```python
from build123d import *

# Parameters (mm, degrees)
F0_W          = 12
F0_H          = 23
F1_DEPTH      = 23.35
F2_W          = 12
F2_H          = 2.3
F3_DEPTH      = 5
F3_DEPTH_BACK = 28
F5_DEPTH      = 3.8
F6_R          = 2.325
F7_DEPTH      = 2.5
F9_DEPTH      = 25
F11_DEPTH     = 25


with BuildPart() as f1:
    # F0 (on Top) → F1 (new body)
    with BuildSketch(Plane.XY):
        Rectangle(F0_W, F0_H)
    extrude(amount=F1_DEPTH)

    # F2 (on face) → F3 (join, two sides)
    with BuildSketch(Plane.XZ.offset(11.5)) as f3_sk:
        with Locations((0, 17.5)):
            Rectangle(F2_W, F2_H)
    extrude(amount=F3_DEPTH)
    extrude(f3_sk.sketch, amount=-F3_DEPTH_BACK)

    # F4 (on face) → F5 (join)
    with BuildSketch(Plane.XY.offset(23.35)):
        with BuildLine():
            ThreePointArc((5.675, 5.825), (4.0128309832, 9.8378309832), (0, 11.5))
            Line((0, 11.5), (0, 5.825))
            Line((0, 5.825), (0, 2.025))
            ThreePointArc((0, 2.025), (1.3761840956, 1.6671324113), (2.4037015124, 0.6841981132))
            ThreePointArc((2.4037015124, 0.6841981132), (4.7878299407, 2.7783117228), (5.675, 5.825))
        make_face()
        with BuildLine():
            Line((0, 5.825), (0, 11.5))
            ThreePointArc((0, 11.5), (-5.5398409592, 7.0561730773), (-2.4037015124, 0.6841981132))
            ThreePointArc((-2.4037015124, 0.6841981132), (-1.3761840956, 1.6671324113), (0, 2.025))
            Line((0, 2.025), (0, 5.825))
        make_face()
        with BuildLine():
            ThreePointArc((0, 2.025), (-1.3761840956, 1.6671324113), (-2.4037015124, 0.6841981132))
            ThreePointArc((-2.4037015124, 0.6841981132), (-1.2311730773, 0.2851590408), (0, 0.15))
            Line((0, 0.15), (0, 2.025))
        make_face()
        with BuildLine():
            ThreePointArc((0, 0.15), (-1.2311730773, 0.2851590408), (-2.4037015124, 0.6841981132))
            ThreePointArc((-2.4037015124, 0.6841981132), (-0.7714169519, -3.5176351643), (2.825, -0.8))
            ThreePointArc((2.825, -0.8), (2.7176351643, -0.0285830481), (2.4037015124, 0.6841981132))
            ThreePointArc((2.4037015124, 0.6841981132), (1.2311730773, 0.2851590408), (0, 0.15))
        make_face()
        with BuildLine():
            ThreePointArc((2.4037015124, 0.6841981132), (1.3761840956, 1.6671324113), (0, 2.025))
            Line((0, 2.025), (0, 0.15))
            ThreePointArc((0, 0.15), (1.2311730773, 0.2851590408), (2.4037015124, 0.6841981132))
        make_face()
    extrude(amount=F5_DEPTH)

    # F6 (on face) → F7 (join)
    with BuildSketch(Plane.XY.offset(27.15)):
        with Locations((0, 5.825)):
            Circle(F6_R)
    extrude(amount=F7_DEPTH)

    # F8 (on face) → F9 (cut)
    with BuildSketch(Plane.XY.offset(18.65)):
        with BuildLine():
            Line((0.55, 14.9), (-0.55, 14.9))
            ThreePointArc((-0.55, 14.9), (-0.7585725469, 14.0049276511), (0, 13.4860589702))
            ThreePointArc((0, 13.4860589702), (0.5755432217, 13.7244567783), (0.8139410298, 14.3))
            ThreePointArc((0.8139410298, 14.3), (0.7450394508, 14.6277441331), (0.55, 14.9))
        make_face()
        with BuildLine():
            Line((0.55, 16.5), (-0.55, 16.5))
            Line((-0.55, 16.5), (-0.55, 14.9))
            ThreePointArc((-0.55, 14.9), (0, 15.1139410298), (0.55, 14.9))
            Line((0.55, 14.9), (0.55, 16.5))
        make_face()
        with BuildLine():
            ThreePointArc((0.55, 14.9), (0, 15.1139410298), (-0.55, 14.9))
            Line((-0.55, 14.9), (0.55, 14.9))
        make_face()
    extrude(amount=-F9_DEPTH, mode=Mode.SUBTRACT)

    # F10 (on face) → F11 (cut)
    with BuildSketch(Plane.XY.offset(18.65)):
        with BuildLine():
            ThreePointArc((0, -13.4860589702), (-0.7585725469, -14.0049276511), (-0.55, -14.9))
            Line((-0.55, -14.9), (0.55, -14.9))
            ThreePointArc((0.55, -14.9), (0.7450394508, -14.6277441331), (0.8139410298, -14.3))
            ThreePointArc((0.8139410298, -14.3), (0.5755432217, -13.7244567783), (0, -13.4860589702))
        make_face()
        with BuildLine():
            ThreePointArc((0.55, -14.9), (0, -15.1139410298), (-0.55, -14.9))
            Line((-0.55, -14.9), (-0.55, -18.1))
            Line((-0.55, -18.1), (0.55, -18.1))
            Line((0.55, -18.1), (0.55, -14.9))
        make_face()
        with BuildLine():
            Line((0.55, -14.9), (-0.55, -14.9))
            ThreePointArc((-0.55, -14.9), (0, -15.1139410298), (0.55, -14.9))
        make_face()
    extrude(amount=-F11_DEPTH, mode=Mode.SUBTRACT)


solid = f1.part
```
Design review of the part built by this model. Coordinates are the model's own, in mm. A direction names the side the tool comes from. Coordinates: 2 decimals unless noted, no trailing zeros. Order: outer loops, then holes, each group sorted by start corner. A loop starts at its lowest first (then second) coordinate and runs counter-clockwise, first axis right, second up. Notation, with made-up numbers: M 1.5,80.5 L 40.5,80.5 A29 cw 40.5,101.5 Z; hole C 15.5,0.5 d2. An arc over 180 degrees is marked long. Answer as a JSON object with one key per item and string values. Group by question number.
1) Add section C-C, the plane y = -1.5. Write out the cut boundary in (x, z), then the cut area to 3 significant figures.
2) Tool access review of faces 1 (the flat face through (0, 13, 16.35)), 2 (the flat face through (0, -11.5, 8)), 3 (the flat face through (-0.55, -16, 18)): name each direction out of +Z, -Z, +X, -X, +Y, -Y from which nothing blocks a thin tool from reaching the whole face with its end or side.
3) Add section D-D, the plane z = 2. Write out the cut boundary in (x, y), then the cut area to 3 significant figures.
4) Add section A-A, the plane z = 17.5. Write out the cut boundary in (x, y).
5) For pin 1 (6 mm diameter, centred on x = -4, y = -11, fed in from +Z); pin 2 (1.4 mm diameter, centred on x = 2.5, z = 21, fed in from +Y); pin 3 (5.5 mm diameter, centred on x = -2, y = 15, fed in from +Z), all flat-tipped, find the tip position at first contact; note any pin that passes through.
6) Add section B-B, the plane x = -4.5. Write out the cut boundary in (y, z).
7) Mouldability with a two-part tool opening along X and no side actions: class faces 4 (the flat face through (-6, 0, 12)), 5 (the flat face through (0, 11.5, 21)), 6 (the flat face through (0.55, -16, 18)) as pulls with the +X half, pulls with the -X half, needs draft (parallel to the pull), parting line crosses it, or undercut.
8) Wall thickness on L1, parallel to Z at x = 2, y = 12.5; L2, parallel to Z at x = -0.5, y = -5; L3, parallel to Y at x = -1, z = 3: over which ranges is each line inside the solid? List them lowest first.
Computed values:
{
 "1": {"outline": "M -6,0 L 6,0 L 6,23.35 L 2.74,23.35 L 2.74,27.15 L -2.74,27.15 L -2.74,23.35 L -6,23.35 Z", "area": "301 mm^2"},
 "2": {"face 1": "-Z, +X, -X, +Y", "face 2": "-Z, +X, -X, -Y", "face 3": "+Z, -Z, -Y"},
 "3": {"outline": "M -6,-11.5 L 6,-11.5 L 6,11.5 L -6,11.5 Z", "area": "276 mm^2"},
 "4": {"outline": "M -6,-16.5 L -0.55,-16.5 L -0.55,-14.9 A0.81 cw long 0.55,-14.9 L 0.55,-16.5 L 6,-16.5 L 6,16.5 L 0.55,16.5 L 0.55,14.9 A0.81 cw long -0.55,14.9 L -0.55,16.5 L -6,16.5 Z"},
 "5": {"pin 1": "stops at z = 23.35", "pin 2": "stops at y = 11.5", "pin 3": "stops at z = 18.65"},
 "6": {"outline": "M -16.5,16.35 L -11.5,16.35 L -11.5,0 L 11.5,0 L 11.5,16.35 L 16.5,16.35 L 16.5,18.65 L 11.5,18.65 L 11.5,23.35 L 9.28,23.35 L 9.28,27.15 L 2.37,27.15 L 2.37,23.35 L -11.5,23.35 L -11.5,18.65 L -16.5,18.65 Z"},
 "7": {"face 4": "pulls with the -X half", "face 5": "needs draft", "face 6": "undercut"},
 "8": {"L1": "z = 16.35 to 18.65", "L2": "z = 0 to 23.35", "L3": "y = -11.5 to 11.5"}
}
